Build history of the part. All positions in model axes, mm. Give positions to 0.01 mm unless a question says otherwise; leave off trailing zeros. Order: outer loops, then holes, each group sorted by start corner. A loop starts at its lowest first (then second) coordinate and runs counter-clockwise, first axis right, second up. Notation, with made-up numbers: (-2, -10.75) - (56, -10.75) arc R25 ccw to (56, 22.25) - close; hole circle Ø5 at (72.5, 21). An arc over 180 degrees is marked (long way). Use a Markdown table: item, result. Add a question column.
(1) Slice it at C-C (z = -2.5). Write the cut outline in (x, y) (1 decimal), then the cut area to 3 significant figures.
(2) Slice it at A-A (y = 0). Write the cut outline in (x, z), then the cut area to 3 significant figures.
(3) Slice it at B-B (z = 4). Write the cut outline in (x, y) (1 decimal), then the cut area to 3 significant figures.
(4) Wall check: line 1 (Y direction, x = 4.75, z = 2.25); line 2 (Y direction, x = 0.25, z = 4.25); line 3 (X direction, y = 2.5, z = 2.25). Give the ranges that are in metal, low to high.
(5) Flat gauge pins, fed straight in: pin 1 (2 mm diameter, centred on x = 5, z = -1.5, fed in from +Y); pin 2 (5 mm diameter, centred on x = -2.5, y = 3, fed in from +Z); pin 3 (4 mm diameter, centred on x = -4.5, z = 2.5, fed in from +Y); pin 4 (2 mm diameter, centred on x = -6.5, z = -2.5, fed in from -Y). Where does each tip first touch, or does it go through?
(6) Mould opens along X. For faces 1 (the face through (-5.885, 10.387, 0.067)), 2 (the face through (7.571, 2.384, -0.061)), 3 (the face through (11.938, 0, 0)) say: +X half, -X half, draft (parallel to the pull), parting line (faces both ways), or undercut.
from build123d import *

# Parameters (mm, degrees)
SKETCH1_R      = 7.9375
EXTRUDE1_DEPTH = 4.826


with BuildPart() as part:
    # Sketch1 → Extrude1 (new body, symmetric)
    with BuildSketch(Plane.XY):
        Polygon((0, 13.784815027), (-11.938, 6.892407514), (-11.938, -6.892407514), (0, -13.784815027), (11.938, -6.892407514), (11.938, 6.892407514), align=None)
        Circle(SKETCH1_R, mode=Mode.SUBTRACT)
    extrude(amount=EXTRUDE1_DEPTH, both=True)

    # Sketch2 → Detail (revolve, cut)
    with BuildSketch(Plane(origin=(0, 0, 0), x_dir=(0, 0, -1), z_dir=(1, 0, 0))):
        Polygon((4.826, 7.9375), (4.826, 8.4375), (4.326, 7.9375), align=None)
        with BuildLine():
            Line((4.826, 13.784815027), (4.826, 11.784815027))
            ThreePointArc((4.826, 11.784815027), (4.240213562, 13.19902859), (2.826, 13.784815027))
            Line((2.826, 13.784815027), (4.826, 13.784815027))
        make_face()
        with BuildLine():
            Line((-2.826, 13.784815027), (-4.826, 13.784815027))
            Line((-4.826, 13.784815027), (-4.826, 11.784815027))
            ThreePointArc((-4.826, 11.784815027), (-4.240213562, 13.19902859), (-2.826, 13.784815027))
        make_face()
        Polygon((-4.326, 7.9375), (-4.826, 7.9375), (-4.826, 8.4375), align=None)
    revolve(axis=Axis((0, 0, 0), (0, 0, -1)), mode=Mode.SUBTRACT)


solid = part.part
Solution:
| question | item | result |
|---|---|---|
| 1 | outline | (-11.9, -6.9) - (0, -13.8) - (11.9, -6.9) - (11.9, 6.9) - (0, 13.8) - (-11.9, 6.9) - close; hole circle Ø15.9 at (0, 0) |
| 1 | area | 296 mm2 |
| 2 | outline | (-11.94, -4.82) arc R2 ccw to (-11.78, -4.83) - (-8.44, -4.83) - (-7.94, -4.33) - (-7.94, 4.33) - (-8.44, 4.83) - (-11.78, 4.83) arc R2 ccw to (-11.94, 4.82) - close; (7.94, -4.33) - (8.44, -4.83) - (11.78, -4.83) arc R2 ccw to (11.94, -4.82) - (11.94, 4.82) arc R2 ccw to (11.78, 4.83) - (8.44, 4.83) - (7.94, 4.33) - close |
| 2 | area | 76.7 mm2 |
| 3 | outline | (-11.9, -6.1) arc R13.4 ccw to (-11.2, -7.3) - (-0.7, -13.4) arc R13.4 ccw to (0.7, -13.4) - (11.2, -7.3) arc R13.4 ccw to (11.9, -6.1) - (11.9, 6.1) arc R13.4 ccw to (11.2, 7.3) - (0.7, 13.4) arc R13.4 ccw to (-0.7, 13.4) - (-11.2, 7.3) arc R13.4 ccw to (-11.9, 6.1) - close; hole circle Ø15.9 at (0, 0) |
| 3 | area | 294 mm2 |
| 4 | line 1 | -11.04 to -6.36, 6.36 to 11.04 |
| 4 | line 2 | -13.19 to -7.93, 7.93 to 13.19 |
| 4 | line 3 | -11.94 to -7.53, 7.53 to 11.94 |
| 5 | pin 1 | y = 11.48 |
| 5 | pin 2 | through |
| 5 | pin 3 | y = 12.34 |
| 5 | pin 4 | y = -10.61 |
| 6 | face 1 | -X half |
| 6 | face 2 | undercut |
| 6 | face 3 | +X half |
